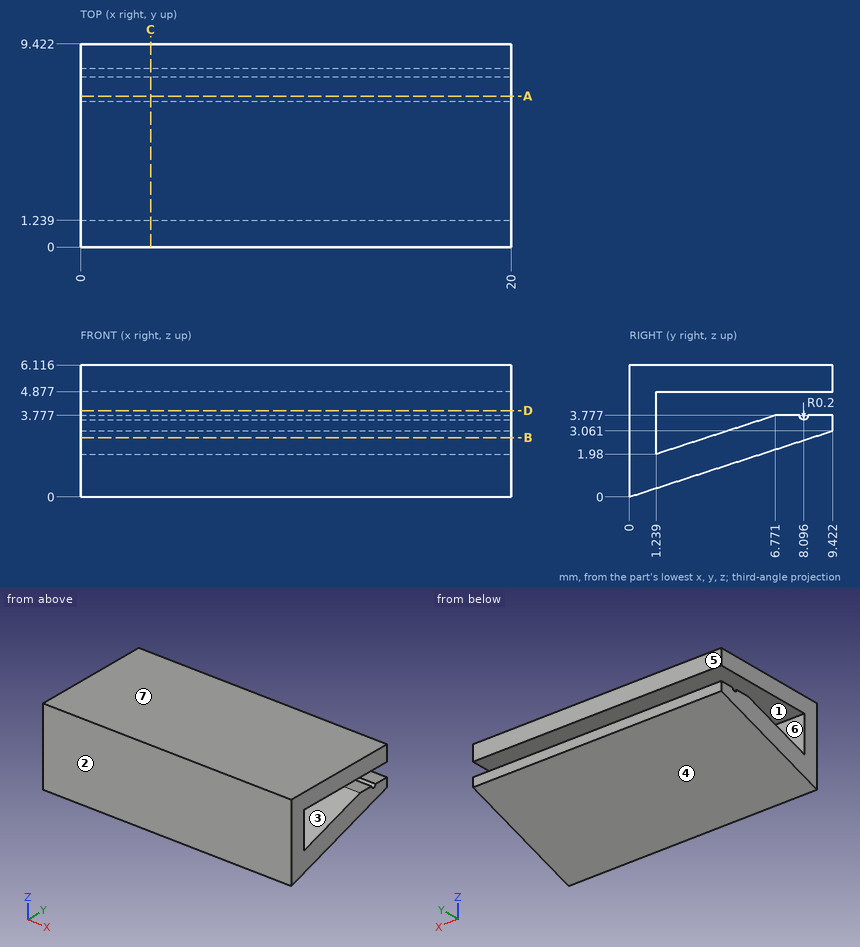
Design review of the part shown in the three views and the two pictorial views. Dimensions are in mm from the part's minimum x, y and z. A direction names the side the tool comes from. Round coordinates to 2 decimals unless told otherwise and drop trailing zeros. Write each loop counter-clockwise with the first axis right and the second up, starting at its lowest first coordinate (ties: lowest second). Pieces come first, ordered by that corner, then holes. Notation, with made-up numbers: (-32, -35) - (14, -35) arc R10 ccw to (14, -20) - close; hole circle Ø11 at (43, -10.75). An arc over 180 degrees is marked (long way). Answer as CSV lines item,"result". Start each with the question number.
(1) Add section A-A, the plane y = 7. State the section outline as (x, z) points (1 decimal).
(2) For pin 1 (2 mm diameter, centred on y = 5, z = 3.5, fed in from -X), flat-tipped, find the tip position at first contact; note if it passes through.
(3) Add section B-B, the plane z = 2.75. State the section outline as (x, y) points, plus the area to 3 significant figures.
(4) Machinability: for the marked faces 1, 2 and 3, which of the approach directions +Z, -Z, +X, -X, +Y, -Y give a long, thin tool a straight path to every point of the face, cutting with its end or side? Answer none if there is none.
(5) Mouldability with a two-part tool opening along Z and no side actions: class the marked faces 4, 5, 6 and 7 as +Z half, -Z half, draft (parallel to the pull), parting line (faces both ways), or undercut.
(6) Add section D-D, the plane z = 4. State the section outline as (x, y) points.
(7) For line 1 (Y direction, x = 2.25, z = 4.5); line 2 (Z direction, x = 4.75, y = 8.5); line 3 (Z direction, x = 8.75, y = 7.25) (1 decimal), list the stretches that pass through material, from the lowest coordinate up.
(8) Add section C-C, the plane x = 3.25. State the section outline as (y, z) points.
From the geometry:
1,outline,"(0, 2.3) - (20, 2.3) - (20, 3.8) - (0, 3.8) - close; (0, 4.9) - (20, 4.9) - (20, 6.1) - (0, 6.1) - close"
2,pin 1,"stops at x = 0"
3,outline,"(0, 0) - (20, 0) - (20, 1.24) - (0, 1.24) - close; (0, 3.61) - (20, 3.61) - (20, 8.46) - (0, 8.46) - close"
3,area,"122 mm²"
4,face 1,"+X, -X, +Y"
4,face 2,"+Z, -Z, +X, -X, -Y"
4,face 3,"+X, -X"
5,face 4,"-Z half"
5,face 5,"draft"
5,face 6,"undercut"
5,face 7,"+Z half"
6,outline,"(0, 0) - (20, 0) - (20, 1.24) - (0, 1.24) - close"
7,line 1,"y = 0 to 1.24"
7,line 2,"z = 2.76 to 3.78, 4.88 to 6.12"
7,line 3,"z = 2.4 to 3.8, 4.9 to 6.1"
8,outline,"(0, 0) - (9.42, 3.06) - (9.42, 3.78) - (8.3, 3.78) arc R0.2 cw to (7.9, 3.78) - (6.77, 3.78) - (1.24, 1.98) - (1.24, 4.88) - (9.42, 4.88) - (9.42, 6.12) - (0, 6.12) - close"
